Answer from the drawing. Dimensions are ordinates in mm from the lowest x, y and z of the part. A direction names the side the tool comes from. Give positions to 0.01 mm unless a question says otherwise; leave off trailing zeros. Write each loop counter-clockwise with the first axis right and the second up, starting at its lowest first coordinate (ties: lowest second). Pieces come first, ordered by that corner, then holes. Notation, with made-up numbers: (58.5, 77.5) -> (84.5, 77.5) arc R28 cw to (84.5, 104.5) -> close; hole circle Ø3 at (70.5, 35.5). An arc over 180 degrees is marked (long way). Use a Markdown table: item, result. Add a question column.
Q1. Each of these flat-tipped pins is pushed along its axis until it touches: pin 1 Ø9.5 at (y, z) = (33, 7.5) entering from +X; pin 2 Ø6.5 at (x, y) = (36.5, 41) entering from +Z; pin 3 Ø5 at (x, y) = (80.5, 31.5) entering from +Z; pin 4 Ø2 at (y, z) = (35, 17.5) entering from +X. Where does it stop, or does it pass through?
Q2. Section D-D, the plane y = 7 is taken. Give the vertices of the cut face in (x, z) (3 decimals).
Q3. Consider line 1 (X direction, y = 25.4, z = 13.5); line 2 (Y direction, x = 38.1, z = 8); line 3 (X direction, y = 25.4, z = 14.5) (3 decimals). Determine where each line is inside the solid, lowest interval first.
Q4. Section A-A, the plane z = 3.5 is taken. Give the vertices of the cut face in (x, y).
Q5. For a pull along X with two mould halves and no side action, classify the marked faces 1, 2, 3 and 4 as pulls with the +X half, pulls with the -X half, needs draft (parallel to the pull), parting line crosses it, or undercut.
Q6. Section C-C, the plane x = 38.1 is taken. Give the vertices of the cut face in (y, z), plus the area to 3 significant figures.
Q7. For the marked faces 5, 6 and 7, determine the directions among +Z, -Z, +X, -X, +Y, -Y from which every point of the face is accessible in a straight line to the end or side of a thin tool.
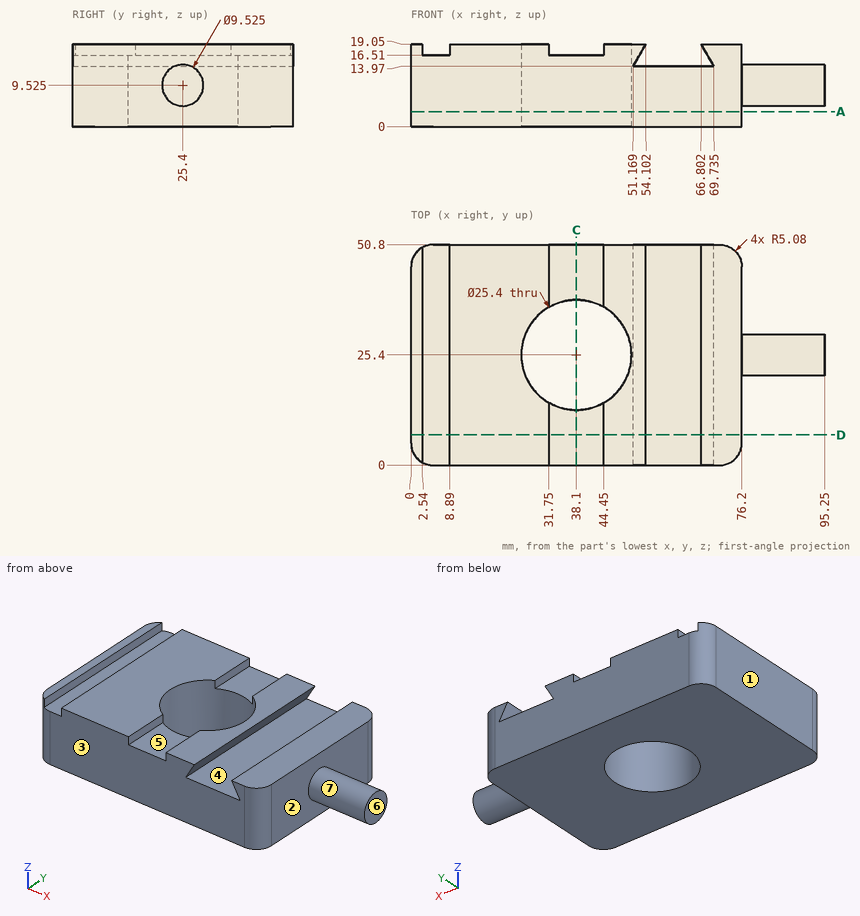
Result set:
| question | item | result |
|---|---|---|
| 1 | pin 1 | stops at x = 95.25 |
| 1 | pin 2 | stops at z = 16.51 |
| 1 | pin 3 | stops at z = 12.64 |
| 1 | pin 4 | stops at x = 76.2 |
| 2 | outline | (0, 0) -> (76.2, 0) -> (76.2, 19.05) -> (66.802, 19.05) -> (69.735, 13.97) -> (51.169, 13.97) -> (54.102, 19.05) -> (44.45, 19.05) -> (44.45, 16.51) -> (31.75, 16.51) -> (31.75, 19.05) -> (8.89, 19.05) -> (8.89, 16.51) -> (2.54, 16.51) -> (2.54, 19.05) -> (0, 19.05) -> close |
| 3 | line 1 | x = 0 to 25.4, 50.8 to 95.25 |
| 3 | line 2 | y = 0 to 12.7, 38.1 to 50.8 |
| 3 | line 3 | x = 0 to 25.4, 50.8 to 51.475, 69.429 to 76.2 |
| 4 | outline | (0, 5.08) arc R5.08 ccw to (5.08, 0) -> (71.12, 0) arc R5.08 ccw to (76.2, 5.08) -> (76.2, 45.72) arc R5.08 ccw to (71.12, 50.8) -> (5.08, 50.8) arc R5.08 ccw to (0, 45.72) -> close; hole circle Ø25.4 at (38.1, 25.4) |
| 5 | face 1 | pulls with the -X half |
| 5 | face 2 | pulls with the +X half |
| 5 | face 3 | needs draft |
| 5 | face 4 | undercut |
| 6 | outline | (0, 0) -> (12.7, 0) -> (12.7, 16.51) -> (0, 16.51) -> close; (38.1, 0) -> (50.8, 0) -> (50.8, 16.51) -> (38.1, 16.51) -> close |
| 6 | area | 419 mm2 |
| 7 | face 5 | +Z, +Y, -Y |
| 7 | face 6 | +Z, -Z, +X, +Y, -Y |
| 7 | face 7 | +X |
